```python
from build123d import *

# Parameters (mm, degrees)
BOSS_EXTRUDE1_DEPTH   = 6
SKETCH2_W             = 10.6165
SKETCH2_H             = 5
BOSS_EXTRUDE2_DEPTH   = 5
CHAMFER1_SIZE         = 2
BOSS_EXTRUDE3_START   = -10
SKETCH3_R             = 4.95
BOSS_EXTRUDE3_DEPTH   = 20
BOSS_EXTRUDE4_START   = 10
SKETCH3_3_R           = 4.95
BOSS_EXTRUDE4_DEPTH   = 10
BOSS_EXTRUDE5_START   = -20
SKETCH3_4_R           = 4.95
BOSS_EXTRUDE5_DEPTH   = 10
F_1_0MM_DOWEL_HOLE1_D = 2.2


with BuildPart() as part:
    # Sketch1 → Boss-Extrude1 (new body)
    with BuildSketch(Plane(origin=(0, 0, 0), x_dir=(1, 0, 0), z_dir=(0, 1, 0))):
        Polygon((16.2325, -10), (10.6165, -10), (5.5005, -10), (5.5005, -20), (16.2325, -20), align=None)
        Polygon((10.6165, 0), (0, 0), (0, -10), (5.5005, -10), (10.6165, -10), align=None)
        Polygon((0, 10), (0, 0), (10.6165, 0), (10.6165, 10), (5.5005, 10), align=None)
        Polygon((5.5005, 10), (10.6165, 10), (16.2325, 10), (16.2325, 20), (5.5005, 20), align=None)
    extrude(amount=BOSS_EXTRUDE1_DEPTH)

    # Sketch2 → Boss-Extrude2 (add)
    with BuildSketch(Plane(origin=(0, 6, 0), x_dir=(1, 0, 0), z_dir=(0, 1, 0))):
        with Locations((5.30825, 7.5)):
            Rectangle(SKETCH2_W, SKETCH2_H)
        with Locations((5.30825, -7.5)):
            Rectangle(SKETCH2_W, SKETCH2_H)
    extrude(amount=BOSS_EXTRUDE2_DEPTH)

    # Chamfer1
    chamfer1_edges = [part.edges().sort_by_distance(p)[0] for p in [
        (5.30825, 11, -5),
        (5.30825, 11, 5),
    ]]
    chamfer(chamfer1_edges, length=CHAMFER1_SIZE)

    # Sketch3 → Boss-Extrude3 (add)
    with BuildSketch(Plane.XY.offset(BOSS_EXTRUDE3_START)):
        with Locations((0, 6.05)):
            Circle(SKETCH3_R)
    extrude(amount=BOSS_EXTRUDE3_DEPTH)

    # Sketch3<3> → Boss-Extrude4 (add)
    with BuildSketch(Plane.XY.offset(BOSS_EXTRUDE4_START)):
        with Locations((16.2325, 6.05)):
            Circle(SKETCH3_3_R)
    extrude(amount=BOSS_EXTRUDE4_DEPTH)

    # Sketch3<4> → Boss-Extrude5 (add)
    with BuildSketch(Plane.XY.offset(BOSS_EXTRUDE5_START)):
        with Locations((16.2325, 6.05)):
            Circle(SKETCH3_4_R)
    extrude(amount=BOSS_EXTRUDE5_DEPTH)

    # Ø1.0mm Dowel Hole1 (through all)
    with Locations(Plane.XY.offset(20)):
        with Locations((0, 6.05), (16.2325, 6.05)):
            Hole(F_1_0MM_DOWEL_HOLE1_D / 2)


solid = part.part
```
Could you check a few things on this model? Use its own coordinates, in mm. A direction names the side the tool comes from. Round coordinates to 2 decimals unless told otherwise and drop trailing zeros. Write each loop counter-clockwise with the first axis right and the second up, starting at its lowest first coordinate (ties: lowest second). Pieces come first, ordered by that corner, then holes.
(1) Suppose I cut it at A-A on z = 2.5. Write out the boundary of the cut face in (x, y).
Findings below:
outline: (0, 0) - (10.62, 0) - (10.62, 6) - (4.95, 6) arc R4.95 ccw (long way) to (0, 1.1) - close; hole circle Ø2.2 at (0, 6.05)
(2) Thinking about a two-plate mould opening in Z: for faces 1 (the face through (13, 4, -20)), 2 (the face through (14.7, 5.6, -10)), 3 (the face through (5, 11, -9)), which applies, +Z half, -Z half, draft (parallel to the pull), parting line (faces both ways), or undercut?
Findings below:
face 1: -Z half
face 2: undercut
face 3: draft
(3) If I drill on probe 1 along Z at (x, y) = (13.75, 7.75); probe 2 along Z at (x, y) = (1.5, 2.75); probe 3 along X at (y, z) = (7.75, 7), over which ranges is the centre line in solid material (lowest first)?
Findings below:
probe 1: z = -20 to -10, 10 to 20
probe 2: z = -10 to 10
probe 3: x = -4.65 to 10.62
(4) Suppose I cut it at C-C on x = 9. Write out the boundary of the cut face in (y, z).
Findings below:
outline: (0, -20) - (6, -20) - (6, -10) - (11, -10) - (11, -7) - (9, -5) - (6, -5) - (6, 5) - (9, 5) - (11, 7) - (11, 10) - (6, 10) - (6, 20) - (0, 20) - close
(5) Suppose I cut it at B-B on x = 12.5. Write out the boundary of the cut face in (y, z), and give its area (3 significant figures).
Findings below:
outline: (0, -20) - (9.3, -20) - (9.3, -10) - (0, -10) - close; (0, 10) - (9.3, 10) - (9.3, 20) - (0, 20) - close
area: 186 mm2
(6) For pin 1 (1 mm diameter, centred on y = 1.5, z = 4.5, fed in from -X); pin 2 (3 mm diameter, centred on x = 7, z = -12.5, fed in from +Y); pin 3 (1.8 mm diameter, centred on y = 2.5, z = -17.5, fed in from -X); pin 4 (1.3 mm diameter, centred on x = 16.23, y = 6.05, fed in from -Z), each with a flat end and sliding along its axis, tell me the tip position at first contact or that it passes through.
Findings below:
pin 1: stops at x = -2.85
pin 2: stops at y = 6
pin 3: stops at x = 5.5
pin 4: passes through
(7) Suppose I cut it at D-D on y = 8.5. Write out the boundary of the cut face in (x, z), and give its area (3 significant figures).
Findings below:
outline: (-4.3, -10) - (10.62, -10) - (10.62, -5) - (4.3, -5) - (4.3, 5) - (10.62, 5) - (10.62, 10) - (-4.3, 10) - close; (11.93, -20) - (20.53, -20) - (20.53, -10) - (11.93, -10) - close; (11.93, 10) - (20.53, 10) - (20.53, 20) - (11.93, 20) - close
area: 407 mm2
(8) Which directions (+Z, -Z, +X, -X, +Y, -Y) give clear straight access to the entire face, cutting with the end or side of a thin tool? Please do faces 4 (the face through (7, 7, -5)), 5 (the face through (8, 6, -15)), 6 (the face through (5.5, 3, 15)), 7 (the face through (8, 6, 15)), 8 (the face through (16.233, 0.5, -14.9)).
Findings below:
face 4: +X, +Y
face 5: -Z, -X, +Y
face 6: +Z, -X, +Y, -Y
face 7: +Z, -X, +Y
face 8: +Z, -Z, +X, -Y
